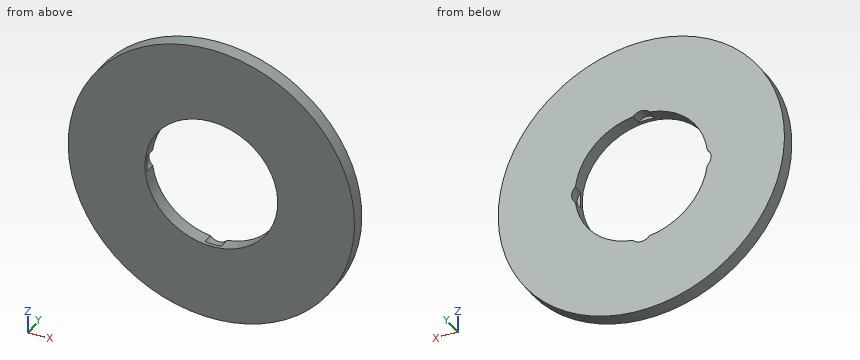
```python
from build123d import *

# Parameters (mm, degrees)
SKETCH1_R           = 70
BOSS_EXTRUDE1_DEPTH = 7
SKETCH2_R           = 32.5
CUT_EXTRUDE1_DEPTH  = 100.242128151
SKETCH3_R           = 5.396472421
CUT_EXTRUDE2_DEPTH  = 5.268712
CIRPATTERN1_START   = 1.731288229
CIRPATTERN1_DEPTH   = 5.268711771


# Read off the part's stored shape, not the designer's step: CirPattern1
with BuildPart() as part:
    # Sketch1 → Boss-Extrude1 (new body)
    with BuildSketch(Plane(origin=(0, 0, 0), x_dir=(1, 0, 0), z_dir=(0, 1, 0))):
        with Locations(Location((0, 0, 0), (0, 0, 270))):
            Circle(SKETCH1_R)
    extrude(amount=BOSS_EXTRUDE1_DEPTH)

    # Sketch2 → Cut-Extrude1 (cut, through all)
    with BuildSketch(Plane(origin=(0, 0, 0), x_dir=(1, 0, 0), z_dir=(0, 1, 0))):
        with Locations(Location((0, 0, 0), (0, 0, 270))):
            Circle(SKETCH2_R)
    extrude(amount=CUT_EXTRUDE1_DEPTH, mode=Mode.SUBTRACT)

    # Sketch3 → Cut-Extrude2 (cut)
    with BuildSketch(Plane(origin=(0, 7, 0), x_dir=(1, 0, 0), z_dir=(0, 1, 0))):
        with Locations((-28.706374574, 0)):
            Circle(SKETCH3_R)
    extrude(amount=-CUT_EXTRUDE2_DEPTH, mode=Mode.SUBTRACT)

    # CirPattern1 outline → CirPattern1 (cut)
    with BuildSketch(Plane(origin=(0, 0, 0), x_dir=(1, 0, 0), z_dir=(0, 1, 0)).offset(CIRPATTERN1_START)):
        with BuildLine():
            ThreePointArc((-4.075677255, 32.24343119), (0, 32.5), (4.075677255, 32.24343119))
            ThreePointArc((4.075677255, 32.24343119), (0, 34.102846995), (-4.075677255, 32.24343119))
        make_face()
        with BuildLine():
            ThreePointArc((32.24343119, -4.075677255), (34.102846995, 0), (32.24343119, 4.075677255))
            ThreePointArc((32.24343119, 4.075677255), (32.5, 0), (32.24343119, -4.075677255))
        make_face()
        with BuildLine():
            ThreePointArc((4.075677255, -32.24343119), (0, -32.5), (-4.075677255, -32.24343119))
            ThreePointArc((-4.075677255, -32.24343119), (0, -34.102846995), (4.075677255, -32.24343119))
        make_face()
    extrude(amount=CIRPATTERN1_DEPTH, mode=Mode.SUBTRACT)


solid = part.part
```
Could you check a few things on this model? Use its own coordinates, in mm. Round coordinates to 2 decimals unless told otherwise and drop trailing zeros. Loops run counter-clockwise (first coordinate to the right, second up) from the corner with the lowest first, then second, coordinate; pieces in that order, holes last.
Q1. For P1, Ø1, axis at y = 6, z = 39, coming from the +X side; P2, Ø0.6, axis at x = 2, z = 33, coming from the +Y side; P3, Ø4, axis at y = 4, z = 4, coming from the -X side, each with a flat end and sliding along its axis, tell me the tip position at first contact or that it passes through.
Q2. I want a section at A-A (z = 0). Write out the boundary of the cut face in (x, y), and give its area (3 significant figures).
Q3. I want a section at B-B (y = 4). Write out the boundary of the cut face in (x, z).
Q4. I want a section at C-C (x = 0). Write out the boundary of the cut face in (y, z), and give its area (3 significant figures).
Q5. I want a section at D-D (z = -20). Write out the boundary of the cut face in (x, y), and give its area (3 significant figures).
Q6. Please list where these lines run through material, in increasing order: L1, parallel to X at y = 6.75, z = 5; L2, parallel to Z at x = 27, y = 3.5; L3, parallel to X at y = 1.25, z = 9.5.
Answer below:
1. P1: stops at x = 58.46
1. P2: stops at y = 1.73
1. P3: stops at x = -69.97
2. outline: (-70, 0) - (-32.5, 0) - (-32.5, 1.73) - (-34.1, 1.73) - (-34.1, 7) - (-70, 7) - close; (32.5, 0) - (70, 0) - (70, 7) - (34.1, 7) - (34.1, 1.73) - (32.5, 1.73) - close
2. area: 508 mm2
3. outline: circle Ø140 at (0, 0); hole (-32.24, -4.08) arc R32.5 ccw to (-4.08, -32.24) arc R5.4 ccw to (4.08, -32.24) arc R32.5 ccw to (32.24, -4.08) arc R5.4 ccw to (32.24, 4.08) arc R32.5 ccw to (4.08, 32.24) arc R5.4 ccw to (-4.08, 32.24) arc R32.5 ccw to (-32.24, 4.08) arc R5.4 ccw to start
4. outline: (0, -70) - (7, -70) - (7, -34.1) - (1.73, -34.1) - (1.73, -32.5) - (0, -32.5) - close; (0, 32.5) - (1.73, 32.5) - (1.73, 34.1) - (7, 34.1) - (7, 70) - (0, 70) - close
4. area: 508 mm2
5. outline: (-67.08, 0) - (-25.62, 0) - (-25.62, 7) - (-67.08, 7) - close; (25.62, 0) - (67.08, 0) - (67.08, 7) - (25.62, 7) - close
5. area: 581 mm2
6. L1: x = -69.82 to -32.11, 32.11 to 69.82
6. L2: z = -64.58 to -18.09, 18.09 to 64.58
6. L3: x = -69.35 to -31.08, 31.08 to 69.35
